```python
from build123d import *

# Parameters (mm, degrees)
EXTRUDE_1_DEPTH = 4.4


with BuildPart() as part:
    # 草图1 → 凸台-拉伸1 (new body)
    with BuildSketch(Plane.XY):
        Polygon((6, 50), (6, 54.4), (-6, 54.4), (-6, 50), (-7, 50), (-12, 50), (-12, 30), (-7, 30), (-7, 10), (-12, 10), (-12, -10), (-7, -10), (-7, -30), (-12, -30), (-12, -50), (-7, -50), (-6, -50), (-6, -54.4), (6, -54.4), (6, -50), (7, -50), (7, -30), (12, -30), (12, -10), (7, -10), (7, 10), (12, 10), (12, 30), (7, 30), (7, 50), align=None)
    extrude(amount=EXTRUDE_1_DEPTH)


solid = part.part
```
Work out the finished part from the listing and answer in its coordinate system (mm). A direction names the side the tool comes from. Round coordinates to 2 decimals unless told otherwise and drop trailing zeros. Order: outer loops, then holes, each group sorted by start corner. A loop starts at its lowest first (then second) coordinate and runs counter-clockwise, first axis right, second up.
Q1. A tool of negligible diameter and unlimited length cuts with its end or side. For faces 4 (the flat face through (7, -40, 2)), 5 (the flat face through (-6, 52, 2)), 6 (the flat face through (10, 30, 2)), 7 (the flat face through (-7, -20, 2)), from which of +Z, -Z, +X, -X, +Y, -Y can it reach the whole face along a straight path? Write none if from no direction.
Solution:
face 4: +Z, -Z, +X, -Y
face 5: +Z, -Z, -X, +Y
face 6: +Z, -Z, +X, +Y
face 7: +Z, -Z, -X
Q2. The mould has two halves that part along Y. Classify faces 1 (the flat face through (-9, -30, 2)), 2 (the flat face through (-12, 40, 2)), 3 (the flat face through (-9, -50, 2)): pulls with the +Y half, pulls with the -Y half, needs draft (parallel to the pull), parting line crosses it, or undercut.
Solution:
face 1: undercut
face 2: needs draft
face 3: pulls with the -Y half
Q3. Given pin 1 Ø2 at (x, z) = (9, 2) entering from -Y; pin 2 Ø1.5 at (x, y) = (-2, -9) entering from -Z; pin 3 Ø2 at (x, z) = (8.5, 3.5) entering from +Y; pin 4 Ø0.5 at (x, z) = (6.5, 2) entering from +Y, each flat-ended and moving along its own axis, determine where each tip first touches the part or whether it passes through.
Solution:
pin 1: stops at y = -30
pin 2: stops at z = 0
pin 3: stops at y = 30
pin 4: stops at y = 50
Q4. A cutting plane is placed at C-C, the plane y = 44. Determine the outline of the cut face in (x, z).
Solution:
outline: (-12, 0) - (7, 0) - (7, 4.4) - (-12, 4.4) - close
Q5. A cutting plane is placed at A-A, the plane x = -9. Determine the outline of the cut face in (y, z), then the cut area to 3 significant figures.
Solution:
outline: (-50, 0) - (-30, 0) - (-30, 4.4) - (-50, 4.4) - close; (-10, 0) - (10, 0) - (10, 4.4) - (-10, 4.4) - close; (30, 0) - (50, 0) - (50, 4.4) - (30, 4.4) - close
area: 264 mm2
Q6. A cutting plane is placed at B-B, the plane z = 2.75. Determine the outline of the cut face in (x, y), then the cut area to 3 significant figures.
Solution:
outline: (-12, -50) - (-6, -50) - (-6, -54.4) - (6, -54.4) - (6, -50) - (7, -50) - (7, -30) - (12, -30) - (12, -10) - (7, -10) - (7, 10) - (12, 10) - (12, 30) - (7, 30) - (7, 50) - (6, 50) - (6, 54.4) - (-6, 54.4) - (-6, 50) - (-12, 50) - (-12, 30) - (-7, 30) - (-7, 10) - (-12, 10) - (-12, -10) - (-7, -10) - (-7, -30) - (-12, -30) - close
area: 2,010 mm2
Q7. Find the intervals of material crossed by line 1 along Y through (x, z) = (-8.75, 2.3); line 2 along Y through (x, z) = (10.5, 2.05); line 3 along X through (y, z) = (7.5, 3.75), in increasing order.
Solution:
line 1: y = -50 to -30, -10 to 10, 30 to 50
line 2: y = -30 to -10, 10 to 30
line 3: x = -12 to 7
